The listing builds one solid part. Answer for the finished solid, in the listing's coordinates (mm). A direction names the side the tool comes from. Give positions to 0.01 mm unless a question says otherwise; leave off trailing zeros. Write each loop counter-clockwise with the first axis right and the second up, starting at its lowest first coordinate (ties: lowest second). Pieces come first, ordered by that corner, then holes. Notation, with made-up numbers: (25.25, 21) - (34.25, 21) arc R19 cw to (34.25, 52) - close; hole circle Ø10 at (6, -17.75). An arc over 180 degrees is marked (long way). Write each question's results on one line, items separated by ' | '. Start each with the question number.
Q1. Section B-B (x = -16) is taken. Determine the outline of the cut face in (y, z), plus the area to 4 significant figures.
Q2. Section D-D (x = 3) is taken. Determine the outline of the cut face in (y, z).
Q3. Flat-ended cylindrical pins translate along their axes: pin 1 Ø1.5 at (x, z) = (-6.5, 0) entering from -Y; pin 2 Ø1 at (y, z) = (-3.5, 4.5) entering from +X; pin 3 Ø4 at (y, z) = (-10.5, 6) entering from -X. Find the tip coordinate at first contact, or state that the pin passes through.
Q4. For a pull along Z with two mould halves and no side action, classify faces 6 (the face through (-7, -19.05, 9)), 7 (the face through (18.146, 1.232, -0.676)), 8 (the face through (-5, -4, -4.08)), 9 (the face through (-4.84, -20.82, 7.02)) as pulls with the +Z half, pulls with the -Z half, needs draft (parallel to the pull), parting line crosses it, or undercut.
Q5. Section C-C (y = -20.25) is taken. Determine the outline of the cut face in (x, z), plus the area to 3 significant figures.
Q6. Section A-A (z = 0) is taken. Determine the outline of the cut face in (x, y) (3 decimals).
Q7. For faces 1 (the face through (-4.841, -22.092, 5.282)), 2 (the face through (-8, -21.55, 9.4)), 3 (the face through (-18.2, 0, 1.5)), 4 (the face through (11, 0, 0)), 5 (the face through (-4.1, -21.55, 9.5)), determine the directions among +Z, -Z, +X, -X, +Y, -Y from which every point of the face is accessible in a straight line to the end or side of a thin tool.
Q8. Find the intervals of material crossed by probe 1 along Z at (x, y) = (-16, 1.6); probe 2 along Z at (x, y) = (-8, -8); probe 3 along X at (y, z) = (-20.25, 4.5), in increasing order.
```python
from build123d import *

# Parameters (mm, degrees)
SKETCH1_W           = 44.45
SKETCH1_H           = 10.16
SKETCH1_R           = 2.25
BOSS_EXTRUDE1_DEPTH = 2.5
SKETCH3_W           = 5
SKETCH3_H           = 10.16
BOSS_EXTRUDE2_DEPTH = 19.05
SKETCH5_W           = 5
SKETCH5_H           = 15.08
SKETCH5_R           = 1.25
BOSS_EXTRUDE3_DEPTH = 2.5
SKETCH6_R           = 2.5
SKETCH6_R_2         = 1.25
BOSS_EXTRUDE4_DEPTH = 1.1
FILLET1_R           = 3.175
CUT_EXTRUDE1_DEPTH  = 1


with BuildPart() as part:
    # Sketch1 → Boss-Extrude1 (new body)
    with BuildSketch(Plane(origin=(0, 0, 0), x_dir=(1, 0, 0), z_dir=(0, 1, 0))):
        Rectangle(SKETCH1_W, SKETCH1_H)
        with Locations((-16, 0)):
            Circle(SKETCH1_R, mode=Mode.SUBTRACT)
        with Locations((16, 0)):
            Circle(SKETCH1_R, mode=Mode.SUBTRACT)
    extrude(amount=BOSS_EXTRUDE1_DEPTH)

    # Sketch3 → Boss-Extrude2 (add)
    with BuildSketch(Plane(origin=(0, 0, 0), x_dir=(-1, 0, 0), z_dir=(0, -1, 0))):
        with Locations((5.9944, 0)):
            Rectangle(SKETCH3_W, SKETCH3_H)
    extrude(amount=BOSS_EXTRUDE2_DEPTH)

    # Sketch5 → Boss-Extrude3 (add)
    with BuildSketch(Plane.XZ.offset(19.05)):
        with Locations((-5.9944, 2.46)):
            Rectangle(SKETCH5_W, SKETCH5_H)
        with Locations((-5.9944, 7.5)):
            Circle(SKETCH5_R, mode=Mode.SUBTRACT)
    extrude(amount=BOSS_EXTRUDE3_DEPTH)

    # Sketch6 → Boss-Extrude4 (add)
    with BuildSketch(Plane.XZ.offset(21.55)):
        with Locations((-5.9944, 7.5)):
            Circle(SKETCH6_R)
        with Locations((-5.9944, 7.5)):
            Circle(SKETCH6_R_2, mode=Mode.SUBTRACT)
    extrude(amount=BOSS_EXTRUDE4_DEPTH)

    # Fillet1
    fillet1_edges = [part.edges().sort_by_distance(p)[0] for p in [
        (-3.4944, 0, 0),
        (-8.4944, 0, 0),
    ]]
    fillet(fillet1_edges, radius=FILLET1_R)

    # Sketch7 → Cut-Extrude1 (cut)
    with BuildSketch(Plane(origin=(0, 0, -5.08), x_dir=(-1, 0, 0), z_dir=(0, 0, -1))):
        with BuildLine():
            Line((-22.225, 0), (0.3194, 0))
            ThreePointArc((0.3194, 0), (2.56446403, -0.92993597), (3.4944, -3.175))
            Line((3.4944, -3.175), (3.4944, -21.55))
            Line((3.4944, -21.55), (8.4944, -21.55))
            Line((8.4944, -21.55), (8.4944, -3.175))
            ThreePointArc((8.4944, -3.175), (9.42433597, -0.92993597), (11.6694, 0))
            Line((11.6694, 0), (22.225, 0))
            Line((22.225, 0), (22.225, 2.5))
            Line((22.225, 2.5), (-22.225, 2.5))
            Line((-22.225, 2.5), (-22.225, 0))
        make_face()
    extrude(amount=-CUT_EXTRUDE1_DEPTH, mode=Mode.SUBTRACT)


solid = part.part
```
Answers below:
1) outline: (0, -4.08) - (2.5, -4.08) - (2.5, -2.25) - (0, -2.25) - close; (0, 2.25) - (2.5, 2.25) - (2.5, 5.08) - (0, 5.08) - close | area: 11.65 mm2
2) outline: (0, -4.08) - (2.5, -4.08) - (2.5, 5.08) - (0, 5.08) - close
3) pin 1: stops at y = -21.55 | pin 2: stops at x = -3.49 | pin 3: stops at x = -8.49
4) face 6: needs draft | face 7: undercut | face 8: pulls with the -Z half | face 9: undercut
5) outline: (-8.49, -4.08) - (-3.49, -4.08) - (-3.49, 10) - (-8.49, 10) - close; hole circle Ø2.5 at (-5.99, 7.5) | area: 65.5 mm2
6) outline: (-22.225, 0) - (-18.25, 0) - (-18.25, 2.5) - (-22.225, 2.5) - close; (-13.75, 0) - (-11.669, 0) arc R3.175 cw to (-8.494, -3.175) - (-8.494, -21.55) - (-3.494, -21.55) - (-3.494, -3.175) arc R3.175 cw to (-0.319, 0) - (13.75, 0) - (13.75, 2.5) - (-13.75, 2.5) - close; (18.25, 0) - (22.225, 0) - (22.225, 2.5) - (18.25, 2.5) - close
7) face 1: -Y | face 2: +Z, -X, -Y | face 3: +Z, -Z, -X, -Y | face 4: +Z, -Z, +X, -Y | face 5: +Z, +X, -Y
8) probe 1: z = -4.08 to -2.25, 2.25 to 5.08 | probe 2: z = -4.08 to 5.08 | probe 3: x = -8.49 to -3.49
